```python
from build123d import *

# Parameters (mm, degrees)
F0_W     = 3
F0_H     = 70
F0_H_2   = 10
F1_DEPTH = 25


with BuildPart() as f1:
    # F0 (on Front) → F1 (new body)
    with BuildSketch(Plane.XZ):
        with BuildLine():
            ThreePointArc((-21.5, 35), (-11.5, 45), (-1.5, 35))
            Line((-1.5, 35), (1.5, 35))
            ThreePointArc((1.5, 35), (-11.5, 48), (-24.5, 35))
            Line((-24.5, 35), (-21.5, 35))
        make_face()
        Rectangle(F0_W, F0_H)
        with Locations((-23, 30)):
            Rectangle(F0_W, F0_H_2)
    extrude(amount=F1_DEPTH)


solid = f1.part
```
Source: CAD feature listing. Evaluate the final solid. Frame: model axes, mm. A direction names the side the tool comes from. Give positions to 0.01 mm unless a question says otherwise; leave off trailing zeros. Order: outer loops, then holes, each group sorted by start corner. A loop starts at its lowest first (then second) coordinate and runs counter-clockwise, first axis right, second up.
(1) Access query for faces 5 (the face through (-24.5, -12, 30)), 6 (the face through (-23, -12, 25)). Directions: +Z, -Z, +X, -X, +Y, -Y. A direction counts if a zero-diameter tool reaches every point of the face in a straight line with its end or side. Return the directions, or none.
(2) Pull-direction query (X, two-part tool) for faces 1 (the face through (1.5, -12, 0)), 2 (the face through (0, -12, -35)), 3 (the face through (-21.5, -12, 30)), 4 (the face through (-11.7, -12.3, 45)); classes: +X half, -X half, draft (parallel to the pull), parting line (faces both ways), or undercut.
(3) Section query A-A (z = 33). Return the cut outline in (x, y), plus the area to 3 significant figures.
(4) Section query B-B (y = -17). Return the cut outline in (x, z).
(5) Section query C-C (z = -7). Return the cut outline in (x, y), plus the area to 3 significant figures.
(6) Material intervals for line 1 along X through (y, z) = (-7.25, 32); line 2 along X through (y, z) = (-6.25, 6); line 3 along Z through (x, y) = (-12, -23.25), sorted ascending.
(7) Section query D-D (x = -18). Return the cut outline in (y, z), plus the area to 3 significant figures.
(8) Contact query for flat-ended pins moving along their axis: P1, Ø1.5, axis at x = -10, y = -8.5, coming from the +Z side; P2, Ø3, axis at y = -8, z = 12, coming from the -X side; P3, Ø4, axis at x = -2, y = -18.5, coming from the +Z side. Output: stop coordinate, or through.
Outcome:
1. face 5: +Z, -Z, -X, +Y, -Y
1. face 6: -Z, -X, +Y, -Y
2. face 1: +X half
2. face 2: draft
2. face 3: undercut
2. face 4: undercut
3. outline: (-24.5, -25) - (-21.5, -25) - (-21.5, 0) - (-24.5, 0) - close; (-1.5, -25) - (1.5, -25) - (1.5, 0) - (-1.5, 0) - close
3. area: 150 mm2
4. outline: (-24.5, 25) - (-21.5, 25) - (-21.5, 35) arc R10 cw to (-1.5, 35) - (-1.5, -35) - (1.5, -35) - (1.5, 35) arc R13 ccw to (-24.5, 35) - close
5. outline: (-1.5, -25) - (1.5, -25) - (1.5, 0) - (-1.5, 0) - close
5. area: 75.0 mm2
6. line 1: x = -24.5 to -21.5, -1.5 to 1.5
6. line 2: x = -1.5 to 1.5
6. line 3: z = 44.99 to 47.99
7. outline: (-25, 42.6) - (0, 42.6) - (0, 46.26) - (-25, 46.26) - close
7. area: 91.5 mm2
8. P1: stops at z = 47.98
8. P2: stops at x = -1.5
8. P3: stops at z = 45.62
